Source: CAD feature listing. Evaluate the final solid. Frame: model axes, mm. A direction names the side the tool comes from. Give positions to 0.01 mm unless a question says otherwise; leave off trailing zeros. Loops run counter-clockwise (first coordinate to the right, second up) from the corner with the lowest first, then second, coordinate; pieces in that order, holes last.
```python
from build123d import *
from OCP.BRepFilletAPI import BRepFilletAPI_MakeChamfer

# Parameters (mm, degrees)
BOSS_EXTRUDE1_DEPTH = 20
CHAMFER1_SIZE       = 10
CHAMFER1_SIZE_2     = 14.838658038
CHAMFER1_SIZE_3     = 8.042998795
SKETCH2_R           = 1
CUT_EXTRUDE1_DEPTH  = 22
SKETCH3_R           = 1
CUT_EXTRUDE2_DEPTH  = 22
CHAMFER2_SIZE       = 2
CHAMFER2_SIZE2      = 2.967731608


with BuildPart() as part:
    # Sketch1 → Boss-Extrude1 (new body)
    with BuildSketch(Plane.XY):
        Polygon((0, 0), (23.377026873, 0), (23.377026873, 4), (-0.166134072, 4), (-0.166134072, 7), (4.755655282, 7), (18.417267614, 7), (4.755655282, 53), (-5.244344718, 53), (-5.244344718, 56), (4.755655282, 56), (4.755655282, 63.7), (-5.244344718, 63.7), (-5.244344718, 66.7), (7.755655282, 66.7), (26.377026873, 4), (26.377026873, -3), (0, -3), align=None)
    extrude(amount=BOSS_EXTRUDE1_DEPTH)

    # Chamfer1
    chamfer1_edges_1 = [part.edges().sort_by_distance(p)[0] for p in [
        (4.755655282, 53, 10),
    ]]
    chamfer1_side_1 = [part.faces().sort_by_distance(p)[0] for p in [
        (4.555655282, 53, 10),
    ]]
    chamfer1_edges_2 = [part.edges().sort_by_distance(p)[0] for p in [
        (18.417267614, 7, 10),
    ]]
    chamfer1_side_2 = [part.faces().sort_by_distance(p)[0] for p in [
        (18.37147062, 7.154203007, 10),
    ]]
    chamfer1 = BRepFilletAPI_MakeChamfer(part.part.solid().wrapped)
    for e in chamfer1_edges_1:
        chamfer1.Add(CHAMFER1_SIZE - 0.0001, CHAMFER1_SIZE_2 - 0.0001, e.wrapped, chamfer1_side_1[0].wrapped)
    for e in chamfer1_edges_2:
        chamfer1.Add(CHAMFER1_SIZE - 0.0001, CHAMFER1_SIZE_3 - 0.0001, e.wrapped, chamfer1_side_2[0].wrapped)
    add(Compound.cast(chamfer1.Shape()), mode=Mode.REPLACE)  # a hair under: the kernel refuses the full size

    # Sketch2 → Cut-Extrude1 (cut)
    with BuildSketch(Plane(origin=(0, 66.7, 0), x_dir=(1, 0, 0), z_dir=(0, 1, 0))):
        with Locations(Location((1.255655282, -10, 0), (0, 0, 180))):
            Circle(SKETCH2_R)
    extrude(amount=-CUT_EXTRUDE1_DEPTH, mode=Mode.SUBTRACT)

    # Sketch3 → Cut-Extrude2 (cut)
    with BuildSketch(Plane(origin=(0, 7, 0), x_dir=(1, 0, 0), z_dir=(0, 1, 0))):
        with Locations(Location((5.104067373, -10, 0), (0, 0, 270))):
            Circle(SKETCH3_R)
    extrude(amount=-CUT_EXTRUDE2_DEPTH, mode=Mode.SUBTRACT)

    # Chamfer2
    chamfer2_edges = [part.edges().sort_by_distance(p)[0] for p in [
        (7.755655282, 66.7, 10),
    ]]
    chamfer2_side = [part.faces().sort_by_distance(p)[0] for p in [
        (17.066341078, 35.35, 10),
    ]]
    chamfer(chamfer2_edges, length=CHAMFER2_SIZE, length2=CHAMFER2_SIZE2, reference=chamfer2_side[0])


solid = part.part
```
(1) Section D-D, the plane z = 10. Count the separate pieces of the cut face and the enclosed holes in it, then the cut area to 3 significant figures.
A:
separate pieces: 5
enclosed holes: 0
area: 693 mm2
(2) First-contact query: pin 1 (3 mm diameter, centred on y = 34, z = 8.5, fed in from -X); pin 2 (2 mm diameter, centred on y = 2, z = 12.5, fed in from -X); pin 3 (10 mm diameter, centred on x = 12, z = 13, fed in from +Y). Flat tips, straight axial feed; report the tip coordinate or a pass-through.
A:
pin 1: stops at x = 9.95
pin 2: stops at x = 23.38
pin 3: stops at y = 65.5
(3) Section B-B, the plane x = 13.5. Return the cut outline in (y, z), then the cut area to 3 significant figures.
A:
outline: (-3, 0) - (0, 0) - (0, 20) - (-3, 20) - close; (4, 0) - (12.77, 0) - (12.77, 20) - (4, 20) - close; (23.56, 0) - (47.36, 0) - (47.36, 20) - (23.56, 20) - close
area: 711 mm2
(4) Reachability of faces 1 (the cylindrical face through (4.496, -1.479, 9.206)), 2 (the flat face through (23.377, 2, 10)), 3 (the flat face through (0, -2, 10)) from +Z, -Z, +X, -X, +Y, -Y: full face, straight path, thin tool, end or side. Return the list, or none.
A:
face 1: -Y
face 2: +Z, -Z, -X
face 3: +Z, -Z, -X, -Y
(5) Section C-C, the plane y = 5.5. Return the cut outline in (x, z).
A:
outline: (-0.17, 0) - (25.93, 0) - (25.93, 20) - (-0.17, 20) - close; hole circle Ø2 at (5.1, 10)
(6) Mould query, pull axis Z, two halves, no side actions, for faces 4 (the flat face through (13, 29, 0)), 5 (the flat face through (0, 56, 10)), 6 (the cylindrical face through (2.255, 50.777, 10.044)), 7 (the cylindrical face through (4.496, 5.521, 9.206)). Classes: pulls with the +Z half, pulls with the -Z half, needs draft (parallel to the pull), parting line crosses it, or undercut.
A:
face 4: pulls with the -Z half
face 5: needs draft
face 6: undercut
face 7: undercut
(7) Ray query, line 1 along Y through (x, z) = (8, 12); line 2 along Y through (x, z) = (3, 3); line 3 along Y through (x, z) = (2, 4). Return the intervals inside material, ascending.
A:
line 1: y = -3 to 0, 4 to 7, 39.76 to 64.96
line 2: y = -3 to 0, 4 to 7, 44.76 to 56, 63.7 to 66.7
line 3: y = -3 to 0, 4 to 7, 45.76 to 56, 63.7 to 66.7
